Geometry check sheet. Reference: the model listing, model coordinates, mm. A direction names the side the tool comes from. Give positions to 0.01 mm unless a question says otherwise; leave off trailing zeros. Loops run counter-clockwise (first coordinate to the right, second up) from the corner with the lowest first, then second, coordinate; pieces in that order, holes last.
1. Cross-section at B-B, the plane z = -366.5. Record the cut outline in (x, y).
2. Release check for a two-part mould opening along X. For faces 3 (the flat face through (-14, -53, -115)), 4 (the flat face through (0, -1, 7)), 5 (the flat face through (-14, 55, 350)) record: +X half, -X half, draft (parallel to the pull), parting line (faces both ways), or undercut.
3. Tool access check on faces 1 (the flat face through (-14, 55, 118)), 2 (the flat face through (-14, 53, 350)). Record the directions out of +Z, -Z, +X, -X, +Y, -Y that give a thin tool (end or side, any length) a straight path to the whole face; none if there is none.
4. Material ranges on L1, parallel to Z at x = -0.9, y = 25; L2, parallel to Y at x = -9, z = 68.5; L3, parallel to X at y = 49.5, z = -40, recorded low to high.
5. Go/stop test with flat-tipped pins: pin 1 Ø3.5 at (x, y) = (-15.5, -52) entering from +Z; pin 2 Ø2 at (x, z) = (-27.5, 232) entering from +Y; pin 3 Ø5 at (y, z) = (-11, 2) entering from -X; pin 4 Ø6 at (x, y) = (-20, -49) entering from -Z. Record where each tip stops, or that it passes through.
6. Cross-section at A-A, the plane x = -10. State how many separate pieces and enclosed holes the cut face has, plus the area to 3 significant figures.
from build123d import *

# Parameters (mm, degrees)
BASE_FLANGE1_DEPTH      = 495
SKETCH6_W               = 30.5
SKETCH6_H               = 20
CUT_EXTRUDE1_DEPTH      = 4.5
LPATTERN1_COUNT         = 3
LPATTERN1_PITCH         = 232.5
LPATTERN1_COL_COUNT     = 3
LPATTERN1_COL_PITCH     = 232.5
MIRROR1_COPY_1_SKETCH_W = 30.5
MIRROR1_COPY_1_SKETCH_H = 20
MIRROR1_COPY_1_DEPTH    = 4.5
MIRROR1_COPY_2_SKETCH_W = 30.5
MIRROR1_COPY_2_SKETCH_H = 20
MIRROR1_COPY_2_DEPTH    = 4.5
MIRROR1_COPY_3_SKETCH_W = 30.5
MIRROR1_COPY_3_SKETCH_H = 20
MIRROR1_COPY_3_DEPTH    = 4.5
MIRROR1_COPY_4_SKETCH_W = 30.5
MIRROR1_COPY_4_SKETCH_H = 20
MIRROR1_COPY_4_DEPTH    = 4.5
CUT_EXTRUDE2_START      = -26
SKETCH7_W               = 40
SKETCH7_H               = 110
CUT_EXTRUDE2_DEPTH      = 26
SKETCH8_W               = 28.862585434
SKETCH8_H               = 32.444228354
SKETCH8_W_2             = 23.227575409
SKETCH8_H_2             = 8.085236505
CUT_EXTRUDE3_DEPTH      = 4.5
CUT_EXTRUDE4_START      = -26
SKETCH9_W               = 93.672664124
SKETCH9_H               = 132.08314216
CUT_EXTRUDE4_DEPTH      = 26
SKETCH10_W              = 25.364032915
SKETCH10_H              = 10.922603619
SKETCH10_W_2            = 22.654683255
SKETCH10_H_2            = 8.37911004
CUT_EXTRUDE5_DEPTH      = 4.5
SKETCH11_R              = 2.75
CUT_EXTRUDE6_DEPTH      = 499.832637264
LPATTERN2_COUNT         = 3
LPATTERN2_PITCH         = 232.5
LPATTERN2_COL_COUNT     = 3
LPATTERN2_COL_PITCH     = 232.5


# Sheet-metal steps are written as plain solids
with BuildPart() as part:
    # Sketch1 → Base-Flange1 (new, symmetric)
    with BuildSketch(Plane.XY):
        with BuildLine():
            Line((-28, -43), (-28, -51.1))
            ThreePointArc((-28, -51.1), (-26.857716447, -53.857716447), (-24.1, -55))
            Line((-24.1, -55), (-3.9, -55))
            ThreePointArc((-3.9, -55), (-1.142283553, -53.857716447), (0, -51.1))
            Line((0, -51.1), (0, 51.1))
            ThreePointArc((0, 51.1), (-1.142283553, 53.857716447), (-3.9, 55))
            Line((-3.9, 55), (-24.1, 55))
            ThreePointArc((-24.1, 55), (-26.857716447, 53.857716447), (-28, 51.1))
            Line((-28, 51.1), (-28, 43))
            Line((-28, 43), (-26, 43))
            Line((-26, 43), (-26, 51.1))
            ThreePointArc((-26, 51.1), (-25.443502884, 52.443502884), (-24.1, 53))
            Line((-24.1, 53), (-3.9, 53))
            ThreePointArc((-3.9, 53), (-2.556497116, 52.443502884), (-2, 51.1))
            Line((-2, 51.1), (-2, -51.1))
            ThreePointArc((-2, -51.1), (-2.556497116, -52.443502884), (-3.9, -53))
            Line((-3.9, -53), (-24.1, -53))
            ThreePointArc((-24.1, -53), (-25.443502884, -52.443502884), (-26, -51.1))
            Line((-26, -51.1), (-26, -43))
            Line((-26, -43), (-28, -43))
        make_face()
    extrude(amount=BASE_FLANGE1_DEPTH, both=True)

    # Sketch6 → Cut-Extrude1 (cut)
    with BuildSketch(Plane(origin=(0, 55, 0), x_dir=(1, 0, 0), z_dir=(0, 1, 0))):
        with Locations((-14, 0)):
            Rectangle(SKETCH6_W, SKETCH6_H)
    cut_extrude1 = extrude(amount=-CUT_EXTRUDE1_DEPTH, mode=Mode.SUBTRACT)

    # LPattern1: Cut-Extrude1 ×3
    with Locations(*[(0, 0, -i * LPATTERN1_PITCH) for i in range(1, LPATTERN1_COUNT)]):
        add(cut_extrude1, mode=Mode.SUBTRACT)

    # LPattern1 col: Cut-Extrude1 ×3
    with Locations(*[(0, 0, i * LPATTERN1_COL_PITCH) for i in range(1, LPATTERN1_COL_COUNT)]):
        add(cut_extrude1, mode=Mode.SUBTRACT)

    # Mirror1: Cut-Extrude1 across plane
    add(cut_extrude1.mirror(Plane.ZX), mode=Mode.SUBTRACT)

    # Mirror1 copy 1 sketch → Mirror1 copy 1 (cut)
    with BuildSketch(Plane(origin=(0, -55, -232.5), x_dir=(1, 0, 0), z_dir=(0, -1, 0))):
        with Locations((-14, 0)):
            Rectangle(MIRROR1_COPY_1_SKETCH_W, MIRROR1_COPY_1_SKETCH_H)
    extrude(amount=-MIRROR1_COPY_1_DEPTH, mode=Mode.SUBTRACT)

    # Mirror1 copy 2 sketch → Mirror1 copy 2 (cut)
    with BuildSketch(Plane(origin=(0, -55, -465), x_dir=(1, 0, 0), z_dir=(0, -1, 0))):
        with Locations((-14, 0)):
            Rectangle(MIRROR1_COPY_2_SKETCH_W, MIRROR1_COPY_2_SKETCH_H)
    extrude(amount=-MIRROR1_COPY_2_DEPTH, mode=Mode.SUBTRACT)

    # Mirror1 copy 3 sketch → Mirror1 copy 3 (cut)
    with BuildSketch(Plane(origin=(0, -55, 232.5), x_dir=(1, 0, 0), z_dir=(0, -1, 0))):
        with Locations((-14, 0)):
            Rectangle(MIRROR1_COPY_3_SKETCH_W, MIRROR1_COPY_3_SKETCH_H)
    extrude(amount=-MIRROR1_COPY_3_DEPTH, mode=Mode.SUBTRACT)

    # Mirror1 copy 4 sketch → Mirror1 copy 4 (cut)
    with BuildSketch(Plane(origin=(0, -55, 465), x_dir=(1, 0, 0), z_dir=(0, -1, 0))):
        with Locations((-14, 0)):
            Rectangle(MIRROR1_COPY_4_SKETCH_W, MIRROR1_COPY_4_SKETCH_H)
    extrude(amount=-MIRROR1_COPY_4_DEPTH, mode=Mode.SUBTRACT)

    # Sketch7 → Cut-Extrude2 (cut)
    with BuildSketch(Plane.ZY.offset(28).offset(CUT_EXTRUDE2_START)):
        with Locations((475, 0)):
            Rectangle(SKETCH7_W, SKETCH7_H)
    extrude(amount=CUT_EXTRUDE2_DEPTH, mode=Mode.SUBTRACT)

    # Sketch8 → Cut-Extrude3 (cut)
    with BuildSketch(Plane(origin=(0, 0, 0), x_dir=(0, 0, -1), z_dir=(1, 0, 0))):
        with Locations((-489.431292717, -66.722114177)):
            Rectangle(SKETCH8_W, SKETCH8_H)
        with Locations((-486.613787705, 54.542618253)):
            Rectangle(SKETCH8_W_2, SKETCH8_H_2)
    extrude(amount=-CUT_EXTRUDE3_DEPTH, mode=Mode.SUBTRACT)

    # Sketch9 → Cut-Extrude4 (cut)
    with BuildSketch(Plane.ZY.offset(28).offset(CUT_EXTRUDE4_START)):
        with Locations((-501.836332062, -11.04157108)):
            Rectangle(SKETCH9_W, SKETCH9_H)
    extrude(amount=CUT_EXTRUDE4_DEPTH, mode=Mode.SUBTRACT)

    # Sketch10 → Cut-Extrude5 (cut)
    with BuildSketch(Plane(origin=(0, 0, 0), x_dir=(0, 0, -1), z_dir=(1, 0, 0))):
        with Locations((487.682016458, -55.96130181)):
            Rectangle(SKETCH10_W, SKETCH10_H)
        with Locations((486.327341628, 54.68955502)):
            Rectangle(SKETCH10_W_2, SKETCH10_H_2)
    extrude(amount=-CUT_EXTRUDE5_DEPTH, mode=Mode.SUBTRACT)

    # Sketch11 → Cut-Extrude6 (cut, through all)
    with BuildSketch(Plane(origin=(0, 0, 0), x_dir=(0, 0, -1), z_dir=(1, 0, 0))):
        with Locations(Location((0, -25, 0), (0, 0, 90))):
            Circle(SKETCH11_R)
        with Locations(Location((0, 25, 0), (0, 0, 90))):
            Circle(SKETCH11_R)
    cut_extrude6 = extrude(amount=-CUT_EXTRUDE6_DEPTH, mode=Mode.SUBTRACT)

    # LPattern2: Cut-Extrude6 ×3
    with Locations(*[(0, 0, -i * LPATTERN2_PITCH) for i in range(1, LPATTERN2_COUNT)]):
        add(cut_extrude6, mode=Mode.SUBTRACT)

    # LPattern2 col: Cut-Extrude6 ×3
    with Locations(*[(0, 0, i * LPATTERN2_COL_PITCH) for i in range(1, LPATTERN2_COL_COUNT)]):
        add(cut_extrude6, mode=Mode.SUBTRACT)


solid = part.part
Result:
1. outline: (-28, -51.1) arc R3.9 ccw to (-24.1, -55) - (-3.9, -55) arc R3.9 ccw to (0, -51.1) - (0, 51.1) arc R3.9 ccw to (-3.9, 55) - (-24.1, 55) arc R3.9 ccw to (-28, 51.1) - (-28, 43) - (-26, 43) - (-26, 51.1) arc R1.9 cw to (-24.1, 53) - (-3.9, 53) arc R1.9 cw to (-2, 51.1) - (-2, -51.1) arc R1.9 cw to (-3.9, -53) - (-24.1, -53) arc R1.9 cw to (-26, -51.1) - (-26, -43) - (-28, -43) - close
2. face 3: undercut
2. face 4: +X half
2. face 5: draft
3. face 1: +Z, -Z, +X, -X, +Y
3. face 2: +Z, -Z
4. L1: z = -495 to -467.75, -462.25 to -235.25, -229.75 to -2.75, 2.75 to 229.75, 235.25 to 462.25, 467.75 to 495
4. L2: y = -55 to -53, 53 to 55
4. L3: x = -28 to -26, -2 to 0
5. pin 1: stops at z = 455
5. pin 2: stops at y = 50.5
5. pin 3: stops at x = -2
5. pin 4: passes through
6. separate pieces: 8
6. enclosed holes: 0
6. area: 3,400 mm2
